Geometry: final body of the model. Coordinates: model frame, mm. A direction names the side the tool comes from. Give positions to 0.01 mm unless a question says otherwise; leave off trailing zeros. Write each loop counter-clockwise with the first axis right and the second up, starting at its lowest first coordinate (ties: lowest second). Pieces come first, ordered by that corner, then holes. Notation, with made-up numbers: (31, -8) -> (54, -8) arc R23 ccw to (54, 20) -> close; hole circle Ø3 at (82, 51.5). An arc over 180 degrees is marked (long way). Answer as a JSON object with one key per item and string values. Group by question number.
(1) Contact query for flat-ended pins moving along their axis: pin 1 Ø5.5 at (y, z) = (25.88, 0) entering from -X; pin 2 Ø3 at (x, y) = (55.5, 22) entering from -Z; pin 3 Ø2 at (y, z) = (24.5, -1.5) entering from +X. Output: stop coordinate, or through.
(2) Material intervals for probe 1 along Y at (x, z) = (57.25, -0.5); probe 2 along X at (y, z) = (27.5, 4); probe 3 along Z at (x, y) = (53, 26.75), sorted ascending.
(3) Section query C-C on x = 60.25. Output: boundary loops of the cut face in (y, z).
(4) Section query B-B on y = 30. Output: boundary loops of the cut face in (x, z), plus the area to 3 significant figures.
(5) Draft query along Y for faces 1 (the face through (54.81, 23, 3)), 2 (the face through (52.431, 23.537, 0.103)), 3 (the face through (61.482, 29.355, 1.093)). Return one class per face: +Y half, -Y half, draft (parallel to the pull), parting line (faces both ways), or undercut.
(6) Set-up query: faces 4 (the face through (56.588, 26, 0)), 5 (the face through (46.854, 28.755, -1.191)), 6 (the face through (43.634, 24, 3)). Return all of +Z, -Z, +X, -X, +Y, -Y with unobstructed straight access to the full face (end or side cutting, diameter ignored); none if empty.
Autodesk Inventor part; units mm, degrees
ref_plane "Work Plane1" through (43.6345, 25.8826, 0) normal (-1, 0, 0) x (0, 0, 1)
ref_plane "YZ Plane" through (0, 0, 0) normal (1, 0, 0) x (0, 1, 0)
ref_plane "XZ Plane" through (0, 0, 0) normal (0, 1, 0) x (-1, 0, 0)
sketch "Sketch1" plane through (0, 0, 0) normal (0, 0, 1) x (1, 0, 0)
  line L0 (56.5885, 25.8826) -> (56.5885, 28.2956)
  line L1 (56.5885, 28.2956) -> (64.9705, 28.2956)
  line L2 (64.9705, 28.2956) -> (64.9705, 29.0576)
  line L3 (64.9705, 29.0576) -> (66.2405, 29.0576)
  line L4 (66.2405, 29.0576) -> (66.2405, 29.5656)
  line L5 (54.153, 29.4566) -> (44.9045, 29.3732)
  line L6 (54.153, 29.4566) -> (54.8105, 29.4566) construction
  line L7 (56.5885, 30.7581) -> (54.8105, 30.7581)
  line L8 (66.2405, 29.5656) -> (56.5885, 29.4785)
  line L9 (54.8105, 29.4625) -> (54.153, 29.4566)
  line L10 (56.5885, 30.7581) -> (56.5885, 29.4785)
  line L11 (54.8105, 30.7581) -> (54.8105, 29.4625)
  line L12 (44.9045, 29.3732) -> (44.9045, 29.6272)
  line L13 (44.9045, 29.6272) -> (43.6345, 29.6272)
  line L14 (43.6345, 29.6272) -> (43.6345, 28.9922)
  line L15 (43.6345, 28.9922) -> (49.9845, 28.9922)
  line L16 (49.9845, 28.9922) -> (49.9845, 28.2302)
  line L17 (49.9845, 28.2302) -> (54.8105, 28.2302)
  line L18 (54.8105, 28.2302) -> (54.8105, 25.8826)
  line L19 (44.9045, 25.8826) -> (67.1022, 25.8826) construction
  line L20 (54.8105, 25.8826) -> (56.5885, 25.8826)
  point P0 (0, 0)
revolve "Revolution1" add sketch "Sketch1" angle 360 about axis through (44.9045, 25.8826, 0) along (1, 0, 0)
ref_plane "Work Plane1" through (43.6345, 25.8826, 0) normal (-1, 0, 0) x (0, 0, 1)
sketch "Sketch5" plane through (43.6345, 25.8826, 0) normal (-1, 0, 0) x (0, 0, 1)
  point P0 (0, -25.8826)
properties part number "AxleTL"
Answer list:
{
 "1": {"pin 1": "x = 49.98", "pin 2": "z = -4.25", "pin 3": "x = 64.97"},
 "2": {"probe 1": "22.32 to 23.52, 28.24 to 29.45", "probe 2": "54.81 to 56.59", "probe 3": "-3.46 to -2.18, 2.18 to 3.46"},
 "3": {"outline": "circle Ø7.26 at (25.88, 0); hole circle Ø4.83 at (25.88, 0)"},
 "4": {"outline": "(54.81, -2.61) -> (56.59, -2.61) -> (56.59, 2.61) -> (54.81, 2.61) -> close", "area": "9.28 mm2"},
 "5": {"face 1": "draft", "face 2": "undercut", "face 3": "parting line"},
 "6": {"face 4": "+X", "face 5": "-X", "face 6": "+Z, -Z, -X, +Y, -Y"}
}
